Verification items for the finished model (mm, model axes). A direction names the side the tool comes from. Give positions to 0.01 mm unless a question says otherwise; leave off trailing zeros. Loops run counter-clockwise (first coordinate to the right, second up) from the corner with the lowest first, then second, coordinate; pieces in that order, holes last. Notation, with made-up numbers: M 43,-13.5 L 63,-13.5 A15 ccw 63,-1.5 Z; hole C 3,11 d11. An arc over 180 degrees is marked long. Write each question's results on one line, items separated by ' | '. Start each with the question number.
```python
from build123d import *

# Parameters (mm, degrees)
F0_W     = 5
F0_H     = 10
F1_DEPTH = 10
F2_W     = 10
F2_H     = 3
F3_DEPTH = 12.7


with BuildPart() as f1:
    # F0 (on Top) → F1 (new body)
    with BuildSketch(Plane.XY):
        with Locations((-15.2, -12.655717)):
            Rectangle(F0_W, F0_H)
    extrude(amount=F1_DEPTH)

    # F2 (on face) → F3 (join, through all)
    with BuildSketch(Plane.YZ.offset(-12.7)):
        with Locations((-12.655717, 8.5)):
            Rectangle(F2_W, F2_H)
    extrude(amount=F3_DEPTH)

    # F4: F1 across plane


with BuildPart() as f1_1:
    add(f1.part)
    add(f1.part.mirror(Plane.YZ))


solid = f1_1.part
```
1. Set-up check for faces 1 (the face through (-12.7, -13, 3)), 2 (the face through (-17.7, -13, 5)): record each of +Z, -Z, +X, -X, +Y, -Y from which the full face is reachable in a straight line by a thin tool's end or side.
2. Thickness scan on probe 1 along X at (y, z) = (-14.75, 3); probe 2 along Z at (x, y) = (3.5, -15). Record the ranges inside material, lowest first.
3. Section check C-C, the plane x = 1.5. Record the boundary of the cut face in (y, z), plus the area to 3 significant figures.
4. Section check A-A, the plane z = 2. Record the boundary of the cut face in (x, y).
5. Section check B-B, the plane y = -13.25. Record the boundary of the cut face in (x, z).
6. Release check for a two-part mould opening along Y. For faces 3 (the face through (0.2, -7.656, 7.2)), 4 (the face through (12.7, -13, 3)), 5 (the face through (0.2, -17.656, 7.2)) record: released by +Y, released by -Y, zero draft, split by the parting line, or undercut.
Filled sheet:
1) face 1: -Z, +Y, -Y | face 2: +Z, -Z, -X, +Y, -Y
2) probe 1: -17.7 to -12.7, 12.7 to 17.7 | probe 2: 7 to 10
3) outline: M -17.66,7 L -7.66,7 L -7.66,10 L -17.66,10 Z | area: 30.0 mm2
4) outline: M -17.7,-17.66 L -12.7,-17.66 L -12.7,-7.66 L -17.7,-7.66 Z; M 12.7,-17.66 L 17.7,-17.66 L 17.7,-7.66 L 12.7,-7.66 Z
5) outline: M -17.7,0 L -12.7,0 L -12.7,7 L 12.7,7 L 12.7,0 L 17.7,0 L 17.7,10 L -17.7,10 Z
6) face 3: released by +Y | face 4: zero draft | face 5: released by -Y
